from build123d import *

# Parameters (mm, degrees)
EXTRUDE_1_DEPTH      = 25
CUT_EXTRUDE_4_DEPTH  = 80.457942189
SKETCH_7_W           = 16.60831278
SKETCH_7_H           = 38.473598513
CUT_EXTRUDE_14_DEPTH = 80.457942189
SKETCH_8_W           = 5
SKETCH_8_H           = 30.968526609
EXTRUDE_2_DEPTH      = 25
SKETCH_9_W           = 2.765387297
SKETCH_9_H           = 65
EXTRUDE_3_DEPTH      = 100
SKETCH_10_W          = 5.026813651
SKETCH_10_H          = 30.968526609
EXTRUDE_4_DEPTH      = 40
CUT_EXTRUDE_15_DEPTH = 100
SKETCH_12_R          = 28.5
CUT_EXTRUDE_16_DEPTH = 100
SKETCH_13_R          = 1.25
CUT_EXTRUDE_17_DEPTH = 100
SKETCH_14_W          = 2.026813651
SKETCH_14_H          = 30.968526609
CUT_EXTRUDE_19_DEPTH = 100
EXTRUDE_5_REACH      = 166.009
SKETCH_16_W          = 2.808181224
SKETCH_16_H          = 99.974557172


with BuildPart() as part:
    # Эскиз1 → Бобышка-Вытянуть1 (new body)
    with BuildSketch(Plane(origin=(0, 0, 0), x_dir=(1, 0, 0), z_dir=(0, 1, 0))):
        Polygon((-66.825757576, 34.969739794), (-66.825757576, 29.969739794), (-63.825757576, 29.969739794), (-63.825757576, 31.969739794), (-38.825757576, 31.969739794), (-38.825757576, 6.969739794), (-63.825757576, 6.969739794), (-63.825757576, 8.969739794), (-66.825757576, 8.969739794), (-66.825757576, 3.969739794), (-22.123470102, 3.969739794), (-36.579007505, 34.969739794), align=None)
    extrude(amount=EXTRUDE_1_DEPTH)

    # Эскиз3 → Вырез-Вытянуть4 (cut, through all)
    with BuildSketch(Plane.XZ):
        Polygon((-66.825757576, -3.969739794), (-65.325757576, -8.969739794), (-66.825757576, -8.969739794), align=None)
        Polygon((-66.825757576, -29.969739794), (-66.825757576, -34.969739794), (-65.325757576, -29.969739794), align=None)
    extrude(amount=-CUT_EXTRUDE_4_DEPTH, mode=Mode.SUBTRACT)

    # Эскиз7 → Вырез-Вытянуть14 (cut, through all)
    with BuildSketch(Plane(origin=(0, 0, 0), x_dir=(-1, 0, 0), z_dir=(0, -1, 0))):
        with Locations((27.703474463, 20.539743139)):
            Rectangle(SKETCH_7_W, SKETCH_7_H)
    extrude(amount=-CUT_EXTRUDE_14_DEPTH, mode=Mode.SUBTRACT)

    # Эскиз8 → Бобышка-Вытянуть2 (add)
    with BuildSketch(Plane(origin=(0, 0, 0), x_dir=(-1, 0, 0), z_dir=(0, -1, 0))):
        with Locations((36.298943925, 19.454003098)):
            Rectangle(SKETCH_8_W, SKETCH_8_H)
    extrude(amount=-EXTRUDE_2_DEPTH)

    # Эскиз9 → Бобышка-Вытянуть3 (add)
    with BuildSketch(Plane(origin=(0, 0, -34.938266403), x_dir=(-1, 0, 0), z_dir=(0, 0, -1))):
        with Locations((38.181637573, 32.5)):
            Rectangle(SKETCH_9_W, SKETCH_9_H)
    extrude(amount=EXTRUDE_3_DEPTH)

    # Эскиз10 → Бобышка-Вытянуть4 (add)
    with BuildSketch(Plane(origin=(0, 25, 0), x_dir=(1, 0, 0), z_dir=(0, 1, 0))):
        with Locations((-36.312350751, 19.454003098)):
            Rectangle(SKETCH_10_W, SKETCH_10_H)
    extrude(amount=EXTRUDE_4_DEPTH)

    # Эскиз11 → Вырез-Вытянуть15 (cut)
    with BuildSketch(Plane(origin=(-33.798943925, 0, 0), x_dir=(0, 0, -1), z_dir=(1, 0, 0))):
        Polygon((34.938266403, 65), (3.969739794, 32.5), (3.969739794, 65), align=None)
    extrude(amount=-CUT_EXTRUDE_15_DEPTH, mode=Mode.SUBTRACT)

    # Эскиз12 → Вырез-Вытянуть16 (cut)
    with BuildSketch(Plane(origin=(-36.798943925, 0, 0), x_dir=(0, 0, -1), z_dir=(1, 0, 0))):
        with Locations((102.438266403, 32.5)):
            Circle(SKETCH_12_R)
    extrude(amount=-CUT_EXTRUDE_16_DEPTH, mode=Mode.SUBTRACT)

    # Эскиз13 → Вырез-Вытянуть17 (cut)
    with BuildSketch(Plane(origin=(-36.798943925, 0, 0), x_dir=(0, 0, -1), z_dir=(1, 0, 0))):
        with Locations((77.438266403, 57.5)):
            Circle(SKETCH_13_R)
        with Locations((127.438266403, 57.5)):
            Circle(SKETCH_13_R)
        with Locations((127.438266403, 7.5)):
            Circle(SKETCH_13_R)
        with Locations((77.438266403, 7.5)):
            Circle(SKETCH_13_R)
    extrude(amount=-CUT_EXTRUDE_17_DEPTH, mode=Mode.SUBTRACT)

    # Эскиз14 → Вырез-Вытянуть19 (cut)
    with BuildSketch(Plane.XZ):
        with Locations((-34.812350751, -19.454003098)):
            Rectangle(SKETCH_14_W, SKETCH_14_H)
    extrude(amount=-CUT_EXTRUDE_19_DEPTH, mode=Mode.SUBTRACT)

    # Бобышка-Вытянуть5: up to this face of the body (flat: up to its plane)
    extrude_5_end = Plane(part.part.faces().sort_by_distance((-38.181637574, 65, -84.938266403))[0])
    # Эскиз16 → Бобышка-Вытянуть5 (add, up to the picked face)
    with BuildSketch(Plane.XZ, mode=Mode.PRIVATE) as extrude_5_sk1:
        with Locations((-40.968421834, -84.95701838)):
            Rectangle(SKETCH_16_W, SKETCH_16_H)
    extrude_5_tool1 = split(extrude(extrude_5_sk1.sketch, amount=-EXTRUDE_5_REACH, mode=Mode.PRIVATE), bisect_by=extrude_5_end, keep=Keep.BOTH, mode=Mode.PRIVATE)
    add(extrude_5_tool1.solids().sort_by(Axis((-40.968422, 0, -84.957018), (0, 1, 0)))[0])


solid = part.part
Could you check a few things on this model? Use its own coordinates, in mm. A direction names the side the tool comes from. Give positions to 0.01 mm unless a question says otherwise; leave off trailing zeros. Order: outer loops, then holes, each group sorted by start corner. A loop starts at its lowest first (then second) coordinate and runs counter-clockwise, first axis right, second up. Notation, with made-up numbers: (-39, 80) -> (-30, 80) arc R12 ccw to (-30, 93) -> close; hole circle Ø7 at (-7, 80). An arc over 180 degrees is marked (long way). Answer in a Markdown table with one row per item. Add a question column.
Item 1: I'm going to push flat-ended pins straight in: P1, Ø4, axis at x = -44.5, y = 35, coming from the -Z side; P2, Ø3, axis at y = 11, z = -51, coming from the -X side; P3, Ø2, axis at x = -41, y = 53, coming from the +Z side; P4, Ø2, axis at y = 7.5, z = -77.44, coming from the +X side. Where does each tip first touch, or does it pass through?
Item 2: For faces 4 (the flat face through (-42.373, 32, -86)), 5 (the flat face through (-39.564, 32, -103)), 6 (the flat face through (-36.799, 32, -73)), 7 (the flat face through (-41, 32, -134.944)), which set-ups out of +Z, -Z, +X, -X, +Y, -Y let a thin tool reach every point of the face, with its end or its side?
Item 3: We'd pull the mould along Z, two halves only. Please class faces 1 (the flat face through (-40, 65, -86)), 2 (the flat face through (-52, 12, -3.97)), 3 (the flat face through (-38.826, 25, -23)): pulls with the +Z half, pulls with the -Z half, needs draft (parallel to the pull), parting line crosses it, or undercut.
Item 4: Imagine slicing it at C-C (z = -59.5). List the corners of the cut face in (x, y) for me, and give its area (3 significant figures).
Item 5: Please list where these lines run through material, in increasing order: probe 1 along Z at (x, y) = (-47.5, 17); probe 2 along X at (y, z) = (17, -101.5); probe 3 along Y at (x, z) = (-39, -34.5).
Item 6: Imagine slicing it at A-A (x = -44.5). List the corners of the cut face in (y, z) for me, and give its area (3 significant figures).
Result:
| question | item | result |
|---|---|---|
| 1 | P1 | through |
| 1 | P2 | x = -42.37 |
| 1 | P3 | z = -34.97 |
| 1 | P4 | x = -39.56 |
| 2 | face 4 | -Z, -X, +Y, -Y |
| 2 | face 5 | +X |
| 2 | face 6 | -Z, +X, +Y, -Y |
| 2 | face 7 | -Z, +X, -X, +Y, -Y |
| 3 | face 1 | needs draft |
| 3 | face 2 | pulls with the +Z half |
| 3 | face 3 | undercut |
| 4 | outline | (-42.37, 0) -> (-36.8, 0) -> (-36.8, 65) -> (-42.37, 65) -> close |
| 4 | area | 362 mm2 |
| 5 | probe 1 | -34.97 to -31.97, -6.97 to -3.97 |
| 5 | probe 2 | -42.37 to -39.56 |
| 5 | probe 3 | 0 to 25 |
| 6 | outline | (0, -34.97) -> (25, -34.97) -> (25, -31.97) -> (0, -31.97) -> close; (0, -6.97) -> (25, -6.97) -> (25, -3.97) -> (0, -3.97) -> close |
| 6 | area | 150 mm2 |
